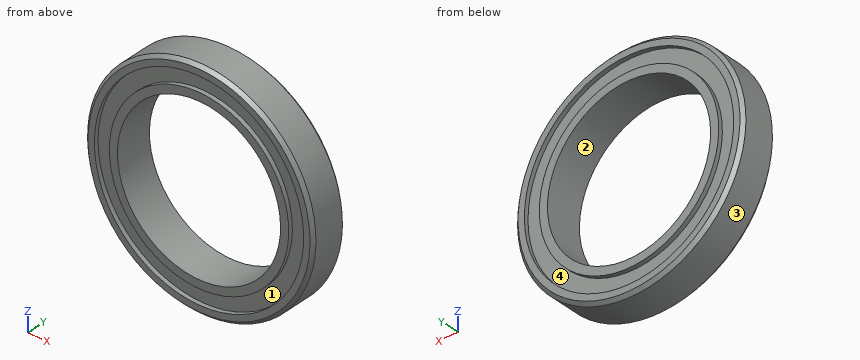
from build123d import *

# Parameters (mm, degrees)
SKETCH_1_R          = 21
SKETCH_1_R_2        = 15
EXTRUDE_1_DEPTH     = 7
CHAMFER_1_SIZE      = 0.6
SKETCH_2_R          = 19.25
SKETCH_2_R_2        = 16.5
CUT_EXTRUDE_1_DEPTH = 0.8
CUT_EXTRUDE_START   = -0.8
SKETCH_3_R          = 19.25
SKETCH_3_R_2        = 16.5
CUT_EXTRUDE_3_DEPTH = 0.8


with BuildPart() as part:
    # 草图1 → 凸台-拉伸1 (new body)
    with BuildSketch(Plane(origin=(0, 0, 0), x_dir=(1, 0, 0), z_dir=(0, 1, 0))):
        with Locations(Location((0, 0, 0), (0, 0, 270))):
            Circle(SKETCH_1_R)
        with Locations(Location((0, 0, 0), (0, 0, 270))):
            Circle(SKETCH_1_R_2, mode=Mode.SUBTRACT)
    extrude(amount=EXTRUDE_1_DEPTH)

    # 倒角1
    chamfer_1_edges = [part.edges().sort_by_distance(p)[0] for p in [
        (0, 0, -21),
        (0, 7, -21),
    ]]
    chamfer(chamfer_1_edges, length=CHAMFER_1_SIZE)

    # 草图2 → 切除-拉伸1 (cut)
    with BuildSketch(Plane(origin=(0, 7, 0), x_dir=(1, 0, 0), z_dir=(0, 1, 0))):
        with Locations(Location((0, 0, 0), (0, 0, 270))):
            Circle(SKETCH_2_R)
        with Locations(Location((0, 0, 0), (0, 0, 270))):
            Circle(SKETCH_2_R_2, mode=Mode.SUBTRACT)
    extrude(amount=-CUT_EXTRUDE_1_DEPTH, mode=Mode.SUBTRACT)

    # 草图3 → 切除-拉伸3 (cut)
    with BuildSketch(Plane.XZ.offset(CUT_EXTRUDE_START)):
        with Locations(Location((0, 0, 0), (0, 0, 90))):
            Circle(SKETCH_3_R)
        with Locations(Location((0, 0, 0), (0, 0, 90))):
            Circle(SKETCH_3_R_2, mode=Mode.SUBTRACT)
    extrude(amount=CUT_EXTRUDE_3_DEPTH, mode=Mode.SUBTRACT)


solid = part.part
Verification items for the finished model (mm, model axes). Face numbers are marked on the shaded views. A direction names the side the tool comes from. Coordinates: 2 decimals unless noted, no trailing zeros. Order: outer loops, then holes, each group sorted by start corner. A loop starts at its lowest first (then second) coordinate and runs counter-clockwise, first axis right, second up. Notation, with made-up numbers: (-19.75, 84.5) -> (1.25, 84.5) arc R5 ccw to (1.25, 88.5) -> close; hole circle Ø3 at (67.25, 26.5). An arc over 180 degrees is marked (long way). Use CSV: the item, a comma, the result in double quotes. Start each with the question number.
Q1. Tool access check on the marked faces 1 and 2. Record the directions out of +Z, -Z, +X, -X, +Y, -Y that give a thin tool (end or side, any length) a straight path to the whole face; none if there is none.
Q2. Draft check along Z on the marked faces 3 and 4. Enter one of: +Z half, -Z half, draft (parallel to the pull), parting line (faces both ways), or undercut.
Q3. Depth check by flat-ended pin: P1, Ø3, axis at x = 10.5, y = 2, coming from the -Z side; P2, Ø2, axis at y = 5.5, z = -10, coming from the +X side; P3, Ø1.5, axis at y = 2, z = -6, coming from the +X side. Enter the tip coordinate at first touch or a pass-through.
Q4. Section check C-C, the plane y = 5.5. Record the cut outline in (x, z).
Q5. Thickness scan on line 1 along X through (y, z) = (0.5, 0); line 2 along X through (y, z) = (6.55, 0); line 3 along X through (y, z) = (5, -1). Record the ranges inside material, lowest first.
Q6. Section check B-B, the plane x = 0. Record the cut outline in (y, z).
Q7. Section check A-A, the plane z = 0. Record the cut outline in (x, y), and give its area (3 significant figures).
Returned:
1,face 1,"-Y"
1,face 2,"+Y, -Y"
2,face 3,"parting line"
2,face 4,"undercut"
3,P1,"stops at z = -18.97"
3,P2,"stops at x = 18.97"
3,P3,"stops at x = 20.33"
4,outline,"circle Ø42 at (0, 0); hole circle Ø30 at (0, 0)"
5,line 1,"x = -20.9 to -19.25, -16.5 to -15, 15 to 16.5, 19.25 to 20.9"
5,line 2,"x = -20.85 to -19.25, -16.5 to -15, 15 to 16.5, 19.25 to 20.85"
5,line 3,"x = -20.98 to -14.97, 14.97 to 20.98"
6,outline,"(0, -20.4) -> (0.6, -21) -> (6.4, -21) -> (7, -20.4) -> (7, -19.25) -> (6.2, -19.25) -> (6.2, -16.5) -> (7, -16.5) -> (7, -15) -> (0, -15) -> (0, -16.5) -> (0.8, -16.5) -> (0.8, -19.25) -> (0, -19.25) -> close; (0, 15) -> (7, 15) -> (7, 16.5) -> (6.2, 16.5) -> (6.2, 19.25) -> (7, 19.25) -> (7, 20.4) -> (6.4, 21) -> (0.6, 21) -> (0, 20.4) -> (0, 19.25) -> (0.8, 19.25) -> (0.8, 16.5) -> (0, 16.5) -> close"
7,outline,"(-21, 0.6) -> (-20.4, 0) -> (-19.25, 0) -> (-19.25, 0.8) -> (-16.5, 0.8) -> (-16.5, 0) -> (-15, 0) -> (-15, 7) -> (-16.5, 7) -> (-16.5, 6.2) -> (-19.25, 6.2) -> (-19.25, 7) -> (-20.4, 7) -> (-21, 6.4) -> close; (15, 0) -> (16.5, 0) -> (16.5, 0.8) -> (19.25, 0.8) -> (19.25, 0) -> (20.4, 0) -> (21, 0.6) -> (21, 6.4) -> (20.4, 7) -> (19.25, 7) -> (19.25, 6.2) -> (16.5, 6.2) -> (16.5, 7) -> (15, 7) -> close"
7,area,"74.5 mm^2"
